Part model, mm, in its own coordinate system. Face numbers are marked on the shaded views. A direction names the side the tool comes from. Round coordinates to 2 decimals unless told otherwise and drop trailing zeros. Loops run counter-clockwise (first coordinate to the right, second up) from the corner with the lowest first, then second, coordinate; pieces in that order, holes last.
from build123d import *

# Parameters (mm, degrees)
SKETCH1_R           = 1.27
BOSS_EXTRUDE1_DEPTH = 1.5875
SKETCH2_R           = 0.79375
CUT_EXTRUDE1_DEPTH  = 1.5875
SKETCH4_W           = 4.7625
SKETCH4_H           = 5.08
BOSS_EXTRUDE2_DEPTH = 3.175


with BuildPart() as part:
    # Sketch1 → Boss-Extrude1 (new body)
    with BuildSketch(Plane(origin=(0, 0, 0), x_dir=(1, 0, 0), z_dir=(0, 1, 0))):
        with BuildLine():
            Line((1.27, 0), (24.13, 0))
            ThreePointArc((24.13, 0), (25.028025612, 0.371974388), (25.4, 1.27))
            Line((25.4, 1.27), (25.4, 16.51))
            ThreePointArc((25.4, 16.51), (25.028025612, 17.408025612), (24.13, 17.78))
            Line((24.13, 17.78), (1.27, 17.78))
            ThreePointArc((1.27, 17.78), (0.371974388, 17.408025612), (0, 16.51))
            Line((0, 16.51), (0, 1.27))
            ThreePointArc((0, 1.27), (0.371974388, 0.371974388), (1.27, 0))
        make_face()
        with Locations((2.54, 15.24)):
            Circle(SKETCH1_R, mode=Mode.SUBTRACT)
        with Locations((22.86, 15.24)):
            Circle(SKETCH1_R, mode=Mode.SUBTRACT)
        with Locations((22.86, 2.54)):
            Circle(SKETCH1_R, mode=Mode.SUBTRACT)
        with Locations((2.54, 2.54)):
            Circle(SKETCH1_R, mode=Mode.SUBTRACT)
    extrude(amount=BOSS_EXTRUDE1_DEPTH)

    # Sketch2 → Cut-Extrude1 (cut)
    with BuildSketch(Plane(origin=(0, 1.5875, 0), x_dir=(1, 0, 0), z_dir=(0, 1, 0))):
        with Locations((6.50875, 15.24)):
            Circle(SKETCH2_R)
        with Locations((8.98525, 15.24)):
            Circle(SKETCH2_R)
        with Locations((11.46175, 15.24)):
            Circle(SKETCH2_R)
        with Locations((13.93825, 15.24)):
            Circle(SKETCH2_R)
        with Locations((16.41475, 15.24)):
            Circle(SKETCH2_R)
        with Locations((18.89125, 15.24)):
            Circle(SKETCH2_R)
        with Locations((6.50875, 2.54)):
            Circle(SKETCH2_R)
        with Locations((8.98525, 2.54)):
            Circle(SKETCH2_R)
        with Locations((11.46175, 2.54)):
            Circle(SKETCH2_R)
        with Locations((13.93825, 2.54)):
            Circle(SKETCH2_R)
        with Locations((16.41475, 2.54)):
            Circle(SKETCH2_R)
        with Locations((18.89125, 2.54)):
            Circle(SKETCH2_R)
    extrude(amount=-CUT_EXTRUDE1_DEPTH, mode=Mode.SUBTRACT)

    # Sketch4 → Boss-Extrude2 (add)
    with BuildSketch(Plane(origin=(0, 1.5875, 0), x_dir=(1, 0, 0), z_dir=(0, 1, 0))):
        with Locations((23.01875, 8.89)):
            Rectangle(SKETCH4_W, SKETCH4_H)
        with Locations((2.38125, 8.89)):
            Rectangle(SKETCH4_W, SKETCH4_H)
    extrude(amount=BOSS_EXTRUDE2_DEPTH)


solid = part.part
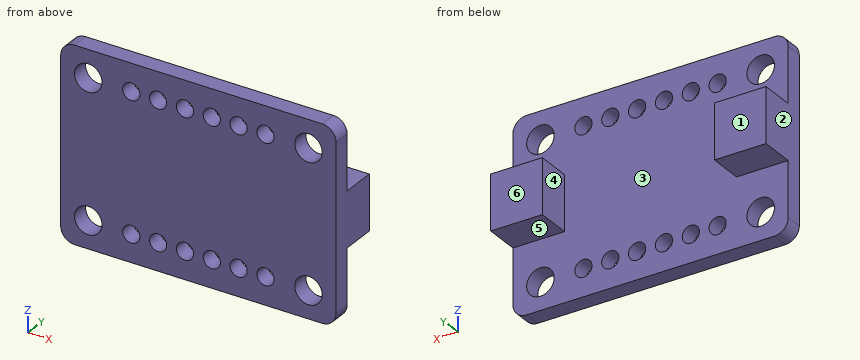
1) Tool access for the marked faces 4, 5 and 6: list every direction of +Z, -Z, +X, -X, +Y, -Y with a clear straight run to the whole face (end or side of a thin tool).
Values:
face 4: +Z, -Z, +Y
face 5: -Z, +X, -X, +Y
face 6: +Z, -Z, +X, -X, +Y
2) Wall check: line 1 along Z through (x, y) = (16.5, 1.5); line 2 along X through (y, z) = (2.1, -10); line 3 along Y through (x, z) = (15.5, -15). Give the ranges that are in metal, low to high.
Values:
line 1: z = -17.78 to -16.03, -14.45 to -3.33, -1.75 to 0
line 2: x = 0 to 4.76, 20.64 to 25.4
line 3: y = 0 to 1.59
3) Mould opens along X. For the marked faces 1, 2 and 3 say: released by +X, released by -X, zero draft, split by the parting line, or undercut.
Values:
face 1: zero draft
face 2: released by -X
face 3: undercut
4) Slice it at D-D, the plane z = -2.54. Give the number of separate pieces and of enclosed holes in the cut face, then the cut area to 3 significant figures.
Values:
separate pieces: 9
enclosed holes: 0
area: 17.1 mm2
5) Slice it at A-A, the plane x = 22.86. Give the cut face in (y, z), then the cut area to 3 significant figures.
Values:
outline: (0, -17.78) - (1.59, -17.78) - (1.59, -16.51) - (0, -16.51) - close; (0, -13.97) - (1.59, -13.97) - (1.59, -11.43) - (4.76, -11.43) - (4.76, -6.35) - (1.59, -6.35) - (1.59, -3.81) - (0, -3.81) - close; (0, -1.27) - (1.59, -1.27) - (1.59, 0) - (0, 0) - close
area: 36.3 mm2
6) Drop flat-ended pins along their axis: pin 1 Ø3 at (x, z) = (18.5, -15) entering from +Y; pin 2 Ø2.5 at (x, y) = (1.5, 3) entering from -Z; pin 3 Ø1 at (x, y) = (2.5, 3.5) entering from +Z. Give the stop position or say it passes through.
Values:
pin 1: stops at y = 1.59
pin 2: stops at z = -11.43
pin 3: stops at z = -6.35
7) Slice it at B-B, the plane y = 3.25. Give the cut face in (x, z), then the cut area to 3 significant figures.
Values:
outline: (0, -11.43) - (4.76, -11.43) - (4.76, -6.35) - (0, -6.35) - close; (20.64, -11.43) - (25.4, -11.43) - (25.4, -6.35) - (20.64, -6.35) - close
area: 48.4 mm2
8) Slice it at C-C, the plane z = -7. Give the cut face in (x, y).
Values:
outline: (0, 0) - (25.4, 0) - (25.4, 4.76) - (20.64, 4.76) - (20.64, 1.59) - (4.76, 1.59) - (4.76, 4.76) - (0, 4.76) - close
